from build123d import *

# Parameters (mm, degrees)
BOSS_EXTRUDE1_DEPTH = 5
BOSS_EXTRUDE2_DEPTH = 15
BOSS_EXTRUDE2_TAPER = 20
SKETCH3_R           = 61
CUT_EXTRUDE1_DEPTH  = 2
SKETCH4_R           = 17
CUT_EXTRUDE2_DEPTH  = 6
CUT_EXTRUDE3_REACH  = 100.658
SKETCH7_R           = 14
SKETCH8_R           = 12.75
CUT_EXTRUDE4_DEPTH  = 16
SKETCH9_R           = 2.1
CUT_EXTRUDE5_DEPTH  = 20
SKETCH12_R          = 4.1
CUT_EXTRUDE7_DEPTH  = 60
SKETCH13_R          = 7.1
CUT_EXTRUDE8_DEPTH  = 18
SKETCH14_W          = 14.5
SKETCH14_H          = 7
CUT_EXTRUDE9_DEPTH  = 16
CUT_EXTRUDE10_START = -5
SKETCH15_R          = 2.1
CUT_EXTRUDE10_DEPTH = 5
CUT_EXTRUDE11_REACH = 101.566
SKETCH16_R          = 6
CUT_EXTRUDE12_DEPTH = 12
CUT_EXTRUDE13_DEPTH = 10


with BuildPart() as part:
    # Sketch1 → Boss-Extrude1 (new body)
    with BuildSketch(Plane(origin=(0, 0, 0), x_dir=(1, 0, 0), z_dir=(0, 1, 0))):
        with BuildLine():
            Line((68.993357168, 12.5), (45.321996131, 53.5))
            ThreePointArc((45.321996131, 53.5), (36.171361037, 62.650635095), (23.671361037, 66))
            Line((23.671361037, 66), (-23.671361037, 66))
            ThreePointArc((-23.671361037, 66), (-36.171361037, 62.650635095), (-45.321996131, 53.5))
            Line((-45.321996131, 53.5), (-68.993357168, 12.5))
            ThreePointArc((-68.993357168, 12.5), (-72.342722074, 0), (-68.993357168, -12.5))
            Line((-68.993357168, -12.5), (-45.321996131, -53.5))
            ThreePointArc((-45.321996131, -53.5), (-36.171361037, -62.650635095), (-23.671361037, -66))
            Line((-23.671361037, -66), (23.671361037, -66))
            ThreePointArc((23.671361037, -66), (36.171361037, -62.650635095), (45.321996131, -53.5))
            Line((45.321996131, -53.5), (68.993357168, -12.5))
            ThreePointArc((68.993357168, -12.5), (72.342722074, 0), (68.993357168, 12.5))
        make_face()
    extrude(amount=BOSS_EXTRUDE1_DEPTH)

    # Sketch2 → Boss-Extrude2 (add)
    with BuildSketch(Plane.XZ):
        with BuildLine():
            Line((-68.993357168, -12.5), (-45.321996131, -53.5))
            ThreePointArc((-45.321996131, -53.5), (-36.171361037, -62.650635095), (-23.671361037, -66))
            Line((-23.671361037, -66), (23.671361037, -66))
            ThreePointArc((23.671361037, -66), (36.171361037, -62.650635095), (45.321996131, -53.5))
            Line((45.321996131, -53.5), (68.993357168, -12.5))
            ThreePointArc((68.993357168, -12.5), (72.342722074, 0), (68.993357168, 12.5))
            Line((68.993357168, 12.5), (45.321996131, 53.5))
            ThreePointArc((45.321996131, 53.5), (36.171361037, 62.650635095), (23.671361037, 66))
            Line((23.671361037, 66), (-23.671361037, 66))
            ThreePointArc((-23.671361037, 66), (-36.171361037, 62.650635095), (-45.321996131, 53.5))
            Line((-45.321996131, 53.5), (-68.993357168, 12.5))
            ThreePointArc((-68.993357168, 12.5), (-72.342722074, 0), (-68.993357168, -12.5))
        make_face()
    extrude(amount=BOSS_EXTRUDE2_DEPTH, taper=BOSS_EXTRUDE2_TAPER)

    # Sketch3 → Cut-Extrude1 (cut)
    with BuildSketch(Plane(origin=(0, 5, 0), x_dir=(1, 0, 0), z_dir=(0, 1, 0))):
        with Locations(Location((0, 0, 0), (0, 0, 270))):
            Circle(SKETCH3_R)
    extrude(amount=-CUT_EXTRUDE1_DEPTH, mode=Mode.SUBTRACT)

    # Sketch4 → Cut-Extrude2 (cut)
    with BuildSketch(Plane(origin=(0, 3, 0), x_dir=(1, 0, 0), z_dir=(0, 1, 0))):
        with Locations(Location((25, 25, 0), (0, 0, 270))):
            Circle(SKETCH4_R)
    extrude(amount=-CUT_EXTRUDE2_DEPTH, mode=Mode.SUBTRACT)

    # Sketch7 → Cut-Extrude3 (cut, up to next)
    with BuildSketch(Plane(origin=(0, -3, 0), x_dir=(1, 0, 0), z_dir=(0, 1, 0)), mode=Mode.PRIVATE) as cut_extrude3_sk1:
        with Locations(Location((25, 25, 0), (0, 0, 270))):
            Circle(SKETCH7_R)
    cut_extrude3_tool1 = extrude(cut_extrude3_sk1.sketch, amount=-CUT_EXTRUDE3_REACH, mode=Mode.PRIVATE) & part.part
    add(cut_extrude3_tool1.solids().sort_by_distance((25, -3, -25))[0], mode=Mode.SUBTRACT)

    # Sketch8 → Cut-Extrude4 (cut)
    with BuildSketch(Plane(origin=(0, -15, 0), x_dir=(-1, 0, 0), z_dir=(0, -1, 0))):
        with Locations(Location((0, 0, 0), (0, 0, 90))):
            Circle(SKETCH8_R)
    extrude(amount=-CUT_EXTRUDE4_DEPTH, mode=Mode.SUBTRACT)

    # Sketch9 → Cut-Extrude5 (cut)
    with BuildSketch(Plane(origin=(0, 3, 0), x_dir=(1, 0, 0), z_dir=(0, 1, 0))):
        with Locations(Location((34, 0, 0), (0, 0, 270))):
            Circle(SKETCH9_R)
        with Locations(Location((-34, 0, 0), (0, 0, 270))):
            Circle(SKETCH9_R)
    extrude(amount=-CUT_EXTRUDE5_DEPTH, mode=Mode.SUBTRACT)

    # Sketch12 → Cut-Extrude7 (cut)
    with BuildSketch(Plane(origin=(0, 0, -66), x_dir=(-1, 0, 0), z_dir=(0, 0, -1))):
        with Locations(Location((0, -7, 0), (0, 0, 90))):
            Circle(SKETCH12_R)
    extrude(amount=-CUT_EXTRUDE7_DEPTH, mode=Mode.SUBTRACT)

    # Sketch13 → Cut-Extrude8 (cut)
    with BuildSketch(Plane(origin=(0, 0, -66), x_dir=(-1, 0, 0), z_dir=(0, 0, -1))):
        with Locations((0, -7)):
            Circle(SKETCH13_R)
    extrude(amount=-CUT_EXTRUDE8_DEPTH, mode=Mode.SUBTRACT)

    # Sketch14 → Cut-Extrude9 (cut)
    with BuildSketch(Plane(origin=(0, -15, 0), x_dir=(-1, 0, 0), z_dir=(0, -1, 0))):
        with Locations((0, 25)):
            Rectangle(SKETCH14_W, SKETCH14_H)
    extrude(amount=-CUT_EXTRUDE9_DEPTH, mode=Mode.SUBTRACT)

    # Sketch15 → Cut-Extrude10 (cut)
    # profile 1 of 2: a face of its own
    with BuildSketch(Plane.XZ.offset(15).offset(CUT_EXTRUDE10_START)):
        Polygon((-34, 4.156921938), (-37.6, 2.078460969), (-37.6, -2.078460969), (-34, -4.156921938), (-30.4, -2.078460969), (-30.4, 2.078460969), align=None)
        with Locations(Location((-34, 0, 0), (0, 0, 90))):
            Circle(SKETCH15_R, mode=Mode.SUBTRACT)
    # profile 2 of 2: a face of its own
    with BuildSketch(Plane.XZ.offset(15).offset(CUT_EXTRUDE10_START)):
        Polygon((34, 4.156921938), (30.4, 2.078460969), (30.4, -2.078460969), (34, -4.156921938), (37.6, -2.078460969), (37.6, 2.078460969), align=None)
        with Locations(Location((34, 0, 0), (0, 0, 90))):
            Circle(SKETCH15_R, mode=Mode.SUBTRACT)
    extrude(amount=CUT_EXTRUDE10_DEPTH, mode=Mode.SUBTRACT)

    # Sketch16 → Cut-Extrude11 (cut, up to next)
    with BuildSketch(Plane(origin=(0, 3, 0), x_dir=(1, 0, 0), z_dir=(0, 1, 0)), mode=Mode.PRIVATE) as cut_extrude11_sk1:
        with Locations(Location((0, -22, 0), (0, 0, 270))):
            Circle(SKETCH16_R)
    cut_extrude11_tool1 = extrude(cut_extrude11_sk1.sketch, amount=-CUT_EXTRUDE11_REACH, mode=Mode.PRIVATE) & part.part
    add(cut_extrude11_tool1.solids().sort_by_distance((0, 3, 22))[0], mode=Mode.SUBTRACT)

    # Sketch17 → Cut-Extrude12 (cut)
    with BuildSketch(Plane(origin=(0, 3, 0), x_dir=(1, 0, 0), z_dir=(0, 1, 0))):
        with BuildLine():
            Line((25, -12), (25, 8))
            ThreePointArc((25, 8), (23.998259334, 8.029539911), (23, 8.118056984))
            Line((23, 8.118056984), (23, -12))
            ThreePointArc((23, -12), (20.656854249, -17.656854249), (15, -20))
            Line((15, -20), (5.656854249, -20))
            ThreePointArc((5.656854249, -20), (5.913591358, -20.985388128), (6, -22))
            Line((6, -22), (15, -22))
            ThreePointArc((15, -22), (22.071067812, -19.071067812), (25, -12))
        make_face()
        with BuildLine():
            ThreePointArc((27, 8.118056984), (26.001740666, 8.029539911), (25, 8))
            Line((25, 8), (25, -12))
            ThreePointArc((25, -12), (22.071067812, -19.071067812), (15, -22))
            Line((15, -22), (6, -22))
            ThreePointArc((6, -22), (5.913591358, -23.014611872), (5.656854249, -24))
            Line((5.656854249, -24), (15, -24))
            ThreePointArc((15, -24), (23.485281374, -20.485281374), (27, -12))
            Line((27, -12), (27, 8.118056984))
        make_face()
        with BuildLine():
            Line((25, 8), (25, 25))
            Line((25, 25), (23, 25))
            Line((23, 25), (23, 8.118056984))
            ThreePointArc((23, 8.118056984), (23.998259334, 8.029539911), (25, 8))
        make_face()
        with BuildLine():
            Line((27, 25), (25, 25))
            Line((25, 25), (25, 8))
            ThreePointArc((25, 8), (26.001740666, 8.029539911), (27, 8.118056984))
            Line((27, 8.118056984), (27, 25))
        make_face()
    extrude(amount=-CUT_EXTRUDE12_DEPTH, mode=Mode.SUBTRACT)

    # Sketch18 → Cut-Extrude13 (cut)
    with BuildSketch(Plane(origin=(0, 3, 0), x_dir=(1, 0, 0), z_dir=(0, 1, 0))):
        with BuildLine():
            Line((5, -25), (5, -45))
            ThreePointArc((5, -45), (0, -50), (-5, -45))
            Line((-5, -45), (-5, -25))
            ThreePointArc((-5, -25), (0, -20), (5, -25))
        make_face()
    extrude(amount=-CUT_EXTRUDE13_DEPTH, mode=Mode.SUBTRACT)


solid = part.part
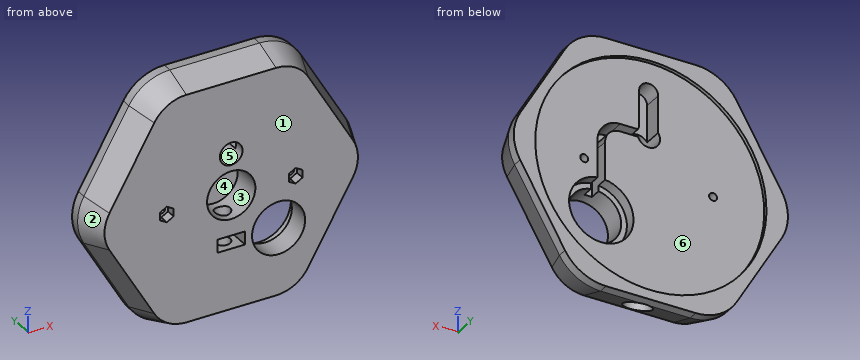
Can you work these out from the model? Positions are in its coordinate system, mm. Face numbers are marked on the shaded views. A direction names the side the tool comes from. Coordinates: 2 decimals unless noted, no trailing zeros. Write item = value, one per line.
(1) I need wall thicknesses on line 1 along X through (y, z) = (-6.5, 1); line 2 along X through (y, z) = (-7, -17.25); line 3 along Z through (x, y) = (-6.5, -4.5). Which ranges of each line are inside material? Lowest first, please. Write a range as [from, to].
Results are:
line_1 = [-69.95, -35.85], [-32.15, -12.71], [12.71, 23], [27, 32.15], [35.85, 69.95]
line_2 = [-63.31, -4.1], [4.1, 13.34], [36.66, 63.31]
line_3 = [-48, -28.5], [-21.5, -10.97], [10.97, 64.36]
(2) For pin 1 Ø2 at (y, z) = (-8.5, -26.5) entering from +X; pin 2 Ø4.5 at (y, z) = (-12, 1) entering from +X; pin 3 Ø7 at (x, y) = (2.5, -7) entering from -Z; pin 4 Ø17 at (x, z) = (25, -25) entering from +Y, each with a flat end and sliding along its axis, tell me the tip position at first contact or that it passes through.
Results are:
pin_1 = 58.05
pin_2 = 68.78
pin_3 = -48
pin_4 = through
(3) If we mould it in two halves opening along X, with no side actions, what happens to the marked faces 1, 2 and 3? For each: pulls with the +X half, pulls with the -X half, needs draft (parallel to the pull), parting line crosses it, or undercut.
Results are:
face_1 = needs draft
face_2 = pulls with the -X half
face_3 = undercut
(4) For the marked faces 4, 5 and 6, which set-ups out of +Z, -Z, +X, -X, +Y, -Y let a thin tool reach every point of the face, with its end or its side?
Results are:
face_4 = -Y
face_5 = +Y, -Y
face_6 = +Y
